Geometry: final body of the model. Coordinates: model frame, mm. A direction names the side the tool comes from. Give positions to 0.01 mm unless a question says otherwise; leave off trailing zeros. Loops run counter-clockwise (first coordinate to the right, second up) from the corner with the lowest first, then second, coordinate; pieces in that order, holes last. Notation, with made-up numbers: (39, 48.25) -> (51, 48.25) arc R10 ccw to (51, 64.25) -> close; hole circle Ø6 at (-3, 80.5). An arc over 180 degrees is marked (long way). One line per question, with ' | ' between items. Start each with the question number.
Item 1: Section C-C on x = 34. Return loops of the section in (y, z), then the cut area to 3 significant figures.
Item 2: Material intervals for line 1 along X through (y, z) = (0, -241); line 2 along Y through (x, z) = (12, 68.5), sorted ascending. Write a range as [from, to].
Item 3: Section D-D on z = -237. Return loops of the section in (x, y), then the cut area to 3 significant figures.
Item 4: Section A-A on y = 0. Return loops of the section in (x, z), then the cut area to 3 significant figures.
Item 5: Pin query (flat end, axial travel): P1, Ø1.5, axis at x = 23.5, z = 56.5, coming from the +Y side; P2, Ø2, axis at x = -58.5, z = 26.5, coming from the +Y side; P3, Ø3, axis at x = 58.5, y = 8, coming from the +Z side; P4, Ø1.5, axis at y = 18, z = -84, coming from the +X side. Return the tip coordinate at first contact, or that it passes through.
Item 6: Mould query, pull axis Y, two halves, no side actions, for faces 3 (the flat face through (57, 10, -266.7)), 4 (the flat face through (60, 0, -177.8)). Classes: released by +Y, released by -Y, zero draft, split by the parting line, or undercut.
Item 7: Set-up query: faces 1 (the flat face through (-60, 0, -177.8)), 2 (the flat face through (0, -58, 177.8)). Return all of +Z, -Z, +X, -X, +Y, -Y with unobstructed straight access to the full face (end or side cutting, diameter ignored); none if empty.
Item 8: Section B-B on z = -55. Return loops of the section in (x, y), then the cut area to 3 significant figures.
from build123d import *

# Parameters (mm, degrees)
BOSS_EXTRUDE1_DEPTH   = 177.8
BOSS_EXTRUDE1_2_DEPTH = 177.8
SKETCH2_R             = 63.5
SKETCH2_R_2           = 57.15
BOSS_EXTRUDE2_DEPTH   = 88.9


with BuildPart() as part:
    # Sketch1 → Boss-Extrude1 (new body, symmetric)
    with BuildSketch(Plane.XY):
        with BuildLine():
            ThreePointArc((60.575139, 19.05), (0, 63.5), (-60.575139, 19.05))
            Line((-60.575139, 19.05), (-53.881537, 19.05))
            ThreePointArc((-53.881537, 19.05), (0, 57.15), (53.881537, 19.05))
            Line((53.881537, 19.05), (60.575139, 19.05))
        make_face()
    extrude(amount=BOSS_EXTRUDE1_DEPTH, both=True)



with BuildPart() as body_2:
    # Sketch1 → Boss-Extrude1 2 (new body, symmetric)
    with BuildSketch(Plane.XY):
        with BuildLine():
            Line((-53.881537, -19.05), (-60.575139, -19.05))
            ThreePointArc((-60.575139, -19.05), (0, -63.5), (60.575139, -19.05))
            Line((60.575139, -19.05), (53.881537, -19.05))
            ThreePointArc((53.881537, -19.05), (0, -57.15), (-53.881537, -19.05))
        make_face()
    extrude(amount=BOSS_EXTRUDE1_2_DEPTH, both=True)


with BuildPart() as part_1:
    add(part.part)

    add(body_2.part)  # Boss-Extrude2 merges body 2
    # Sketch2 → Boss-Extrude2 (add)
    with BuildSketch(Plane(origin=(0, 0, -177.8), x_dir=(-1, 0, 0), z_dir=(0, 0, -1))):
        Circle(SKETCH2_R)
        Circle(SKETCH2_R_2, mode=Mode.SUBTRACT)
    extrude(amount=BOSS_EXTRUDE2_DEPTH)


solid = part_1.part
Result sheet:
1) outline: (-53.63, -266.7) -> (-45.94, -266.7) -> (-45.94, 177.8) -> (-53.63, 177.8) -> close; (45.94, -266.7) -> (53.63, -266.7) -> (53.63, 177.8) -> (45.94, 177.8) -> close | area: 6,840 mm²
2) line 1: x = [-63.5, -57.15], [57.15, 63.5] | line 2: y = [-62.36, -55.88], [55.88, 62.36]
3) outline: circle Ø127 at (0, 0); hole circle Ø114.3 at (0, 0) | area: 2,410 mm²
4) outline: (-63.5, -266.7) -> (-57.15, -266.7) -> (-57.15, -177.8) -> (-63.5, -177.8) -> close; (57.15, -266.7) -> (63.5, -266.7) -> (63.5, -177.8) -> (57.15, -177.8) -> close | area: 1,130 mm²
5) P1: stops at y = 59.28 | P2: stops at y = 26.94 | P3: stops at z = -177.8 | P4: passes through
6) face 3: zero draft | face 4: undercut
7) face 1: +Z, +X, -X | face 2: +Z, +X, -X, +Y, -Y
8) outline: (-60.58, -19.05) arc R63.5 ccw to (60.58, -19.05) -> (53.88, -19.05) arc R57.15 cw to (-53.88, -19.05) -> close; (-60.58, 19.05) -> (-53.88, 19.05) arc R57.15 cw to (53.88, 19.05) -> (60.58, 19.05) arc R63.5 ccw to start | area: 1,910 mm²
